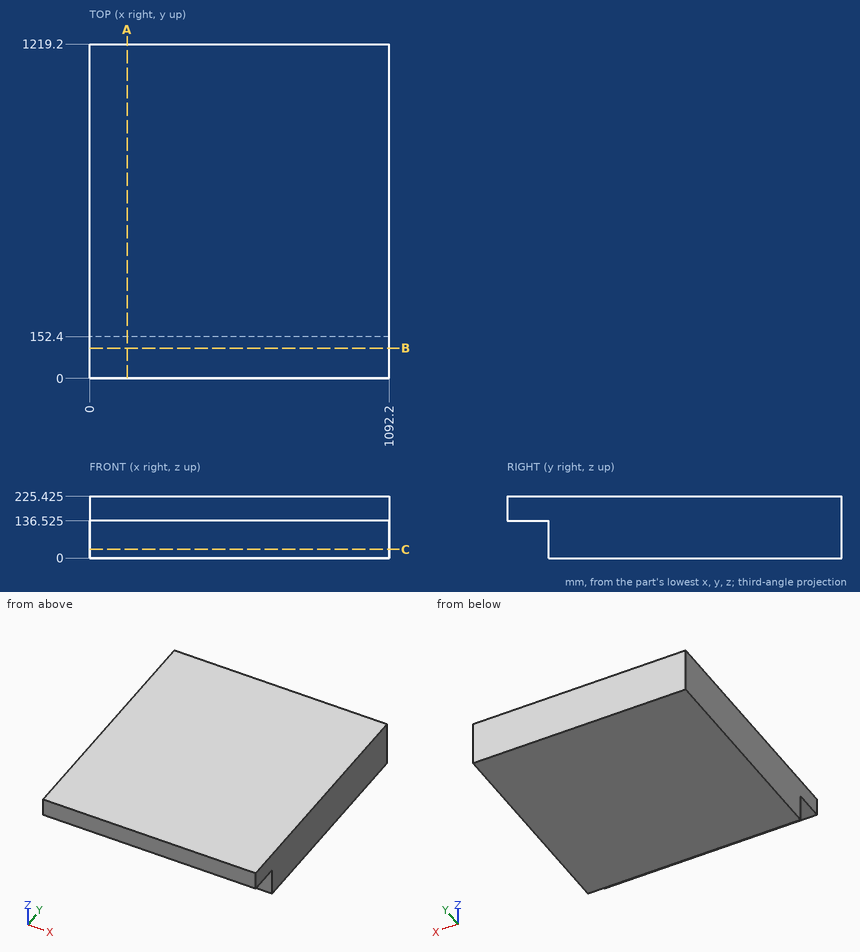
For this review, use the dimensioned drawing (mm, ordinates from the lowest corner) and the shaded views. Round coordinates to 2 decimals unless told otherwise and drop trailing zeros. Order: outer loops, then holes, each group sorted by start corner. A loop starts at its lowest first (then second) coordinate and runs counter-clockwise, first axis right, second up.
1) Consider section A-A (x = 137). State the section outline as (y, z) points (3 decimals).
The answers:
outline: (0, 136.525) - (152.4, 136.525) - (152.4, 0) - (1219.2, 0) - (1219.2, 225.425) - (0, 225.425) - close
2) Consider section C-C (z = 32). State the section outline as (x, y) points.
The answers:
outline: (0, 152.4) - (1092.2, 152.4) - (1092.2, 1219.2) - (0, 1219.2) - close
3) For L1, parallel to Y at x = 543, z = 97, list the stretches that pass through material, from the lowest coordinate up.
The answers:
L1: y = 152.4 to 1219.2
4) Clearance check with a flat-ended pin moving along its axis: pin 1 Ø8 at (x, z) = (838.5, 26) entering from -Y. State where the tip first meets the part, or that it passes through.
The answers:
pin 1: stops at y = 152.4
5) Consider section B-B (y = 110). State the section outline as (x, z) points (3 decimals).
The answers:
outline: (0, 136.525) - (1092.2, 136.525) - (1092.2, 225.425) - (0, 225.425) - close
